```python
from build123d import *

# Parameters (mm, degrees)
F0_R     = 2.5
F0_R_2   = 1.1
F1_DEPTH = 4
F2_R     = 2


with BuildPart() as f1:
    # F0 (on Top) → F1 (new body)
    with BuildSketch(Plane.XY):
        Polygon((7.9, 16.392971), (0, 16.392971), (-7.9, 16.392971), (-7.9, -11.607029), (0, -11.607029), (7.9, -11.607029), align=None)
        with Locations((0, -6.607029)):
            Circle(F0_R, mode=Mode.SUBTRACT)
        with Locations((-4.25, 12.392971)):
            Circle(F0_R_2, mode=Mode.SUBTRACT)
        with Locations((2.25, 12.392971)):
            Circle(F0_R_2, mode=Mode.SUBTRACT)
    extrude(amount=F1_DEPTH)

    # F2
    f2_edges = [f1.edges().sort_by_distance(p)[0] for p in [
        (7.9, -11.607029, 2),
        (7.9, 16.392971, 2),
        (-7.9, -11.607029, 2),
        (-7.9, 16.392971, 2),
    ]]
    fillet(f2_edges, radius=F2_R)


solid = f1.part
```
Work out the finished part from the listing and answer in its coordinate system (mm). Give positions to 0.01 mm unless a question says otherwise; leave off trailing zeros. Write each loop counter-clockwise with the first axis right and the second up, starting at its lowest first coordinate (ties: lowest second). Pieces come first, ordered by that corner, then holes. Notation, with made-up numbers: (-4.75, 35) -> (54.25, 35) arc R24 cw to (54.25, 47) -> close; hole circle Ø11 at (-6, 51.5). An arc over 180 degrees is marked (long way). Write item = value, one per line.
Q1. For a pull along Y with two mould halves and no side action, classify faces 1 (the cylindrical face through (-4.393, 13.484, 1.972)), 2 (the cylindrical face through (-0.54, -9.05, 1.97)), 3 (the flat face through (-7.9, 3, 2)), 4 (the cylindrical face through (-7.3, 15.82, 2.03)) as pulls with the +Y half, pulls with the -Y half, needs draft (parallel to the pull), parting line crosses it, or undercut.
Computed values:
face_1 = undercut
face_2 = undercut
face_3 = needs draft
face_4 = pulls with the +Y half
Q2. Consider line 1 along Y through (x, z) = (-4.25, 1.85); line 2 along X through (y, z) = (12.25, 2); line 3 along Y through (x, z) = (1.5, 1.15). Determine where each line is inside the solid, lowest interval first.
Computed values:
line_1 = -11.61 to 11.29, 13.49 to 16.39
line_2 = -7.9 to -5.34, -3.16 to 1.16, 3.34 to 7.9
line_3 = -11.61 to -8.61, -4.61 to 11.59, 13.2 to 16.39
Q3. Section B-B on z = 0.6 is taken. Determine the outline of the cut face in (x, y), and give its area (3 significant figures).
Computed values:
outline = (-7.9, -9.61) arc R2 ccw to (-5.9, -11.61) -> (5.9, -11.61) arc R2 ccw to (7.9, -9.61) -> (7.9, 14.39) arc R2 ccw to (5.9, 16.39) -> (-5.9, 16.39) arc R2 ccw to (-7.9, 14.39) -> close; hole circle Ø2.2 at (-4.25, 12.39); hole circle Ø5 at (0, -6.61); hole circle Ø2.2 at (2.25, 12.39)
area = 412 mm^2
Q4. A flat-ended cylindrical pin translates along its axis: pin 1 Ø1.3 at (x, y) = (-4.25, 12.39) entering from -Z. Find the tip coordinate at first contact, or state that the pin passes through.
Computed values:
pin_1 = through
Q5. Section A-A on x = 0 is taken. Determine the outline of the cut face in (y, z), and give its area (3 significant figures).
Computed values:
outline = (-11.61, 0) -> (-9.11, 0) -> (-9.11, 4) -> (-11.61, 4) -> close; (-4.11, 0) -> (16.39, 0) -> (16.39, 4) -> (-4.11, 4) -> close
area = 92.0 mm^2
Q6. Section C-C on y = -8.75 is taken. Determine the outline of the cut face in (x, z).
Computed values:
outline = (-7.9, 0) -> (-1.29, 0) -> (-1.29, 4) -> (-7.9, 4) -> close; (1.29, 0) -> (7.9, 0) -> (7.9, 4) -> (1.29, 4) -> close
